from build123d import *

# Parameters (mm, degrees)
SKETCH1_R           = 1.8
BOSS_EXTRUDE1_DEPTH = 3
SKETCH2_R           = 3
SKETCH2_R_2         = 1.8
BOSS_EXTRUDE2_DEPTH = 2


with BuildPart() as part:
    # Sketch1 → Boss-Extrude1 (new body)
    with BuildSketch(Plane(origin=(0, 0, 0), x_dir=(0, 0, -1), z_dir=(1, 0, 0))):
        with BuildLine():
            Line((-66.603258311, 3.562711266), (-16.603258311, 3.562711266))
            ThreePointArc((-16.603258311, 3.562711266), (-13.603258311, 6.562711266), (-16.603258311, 9.562711266))
            Line((-16.603258311, 9.562711266), (-66.603258311, 9.562711266))
            ThreePointArc((-66.603258311, 9.562711266), (-69.603258311, 6.562711266), (-66.603258311, 3.562711266))
        make_face()
        with Locations((-66.603258311, 6.562711266)):
            Circle(SKETCH1_R, mode=Mode.SUBTRACT)
        with Locations((-16.603258311, 6.562711266)):
            Circle(SKETCH1_R, mode=Mode.SUBTRACT)
    extrude(amount=BOSS_EXTRUDE1_DEPTH)

    # Sketch2 → Boss-Extrude2 (add)
    with BuildSketch(Plane(origin=(3, 0, 0), x_dir=(0, 0, -1), z_dir=(1, 0, 0))):
        with Locations((-66.603258311, 6.562711266)):
            Circle(SKETCH2_R)
        with Locations((-66.603258311, 6.562711266)):
            Circle(SKETCH2_R_2, mode=Mode.SUBTRACT)
        with Locations((-16.603258311, 6.562711266)):
            Circle(SKETCH2_R)
        with Locations((-16.603258311, 6.562711266)):
            Circle(SKETCH2_R_2, mode=Mode.SUBTRACT)
    extrude(amount=BOSS_EXTRUDE2_DEPTH)


solid = part.part
Can you work these out from the model? Positions are in its coordinate system, mm. Give positions to 0.01 mm unless a question says otherwise; leave off trailing zeros. Write each loop counter-clockwise with the first axis right and the second up, starting at its lowest first coordinate (ties: lowest second). Pieces come first, ordered by that corner, then holes. Notation, with made-up numbers: M 49,-1 L 63,-1 A32 ccw 63,36 Z; hole C 13,-30.75 d5. An arc over 180 degrees is marked long. Answer in a Markdown table with one row per item. Add a question column.
Item 1: Imagine slicing it at A-A, the plane y = 7.75. Write out the boundary of the cut face in (x, z), plus the area to 3 significant figures.
Item 2: Imagine slicing it at D-D, the plane x = 2.1. Write out the boundary of the cut face in (y, z), plus the area to 3 significant figures.
Item 3: Please list where these lines run through material, in increasing order: L1, parallel to Z at x = 1.3, y = 6.75; L2, parallel to Z at x = 3.35, y = 6.5; L3, parallel to Z at x = 3.35, y = 8.
Item 4: We'd pull the mould along Z, two halves only. Please class faces 1 (the flat face through (1, 3.563, 42)), 2 (the cylindrical face through (3, 6.7, 69.6)), 3 (the cylindrical face through (2.465, 5.147, 13.958)): released by +Z, released by -Z, zero draft, split by the parting line, or undercut.
Item 5: For pin 1 Ø3 at (y, z) = (6.56, 16.6) entering from -X; pin 2 Ø1.5 at (y, z) = (8.5, 20.5) entering from +X; pin 3 Ø3 at (y, z) = (7.5, 34.5) entering from -X, each with a flat end and sliding along its axis, tell me the tip position at first contact or that it passes through.
Item 6: Imagine slicing it at C-C, the plane z = 53. Write out the boundary of the cut face in (x, y), plus the area to 3 significant figures.
Evaluation:
| question | item | result |
|---|---|---|
| 1 | outline | M 0,13.85 L 5,13.85 L 5,15.25 L 0,15.25 Z; M 0,17.96 L 5,17.96 L 5,19.36 L 3,19.36 L 3,63.85 L 5,63.85 L 5,65.25 L 0,65.25 Z; M 0,67.96 L 5,67.96 L 5,69.36 L 0,69.36 Z |
| 1 | area | 162 mm² |
| 2 | outline | M 3.56,16.6 A3 ccw 9.56,16.6 L 9.56,66.6 A3 ccw 3.56,66.6 Z; hole C 6.56,16.6 d3.6; hole C 6.56,66.6 d3.6 |
| 2 | area | 308 mm² |
| 3 | L1 | z = 13.61 to 14.81, 18.39 to 64.81, 68.39 to 69.6 |
| 3 | L2 | z = 13.6 to 14.8, 18.4 to 19.6, 63.6 to 64.8, 68.4 to 69.6 |
| 3 | L3 | z = 13.97 to 15.52, 17.69 to 19.24, 63.97 to 65.52, 67.69 to 69.24 |
| 4 | face 1 | zero draft |
| 4 | face 2 | undercut |
| 4 | face 3 | undercut |
| 5 | pin 1 | passes through |
| 5 | pin 2 | stops at x = 3 |
| 5 | pin 3 | stops at x = 0 |
| 6 | outline | M 0,3.56 L 3,3.56 L 3,9.56 L 0,9.56 Z |
| 6 | area | 18.0 mm² |
